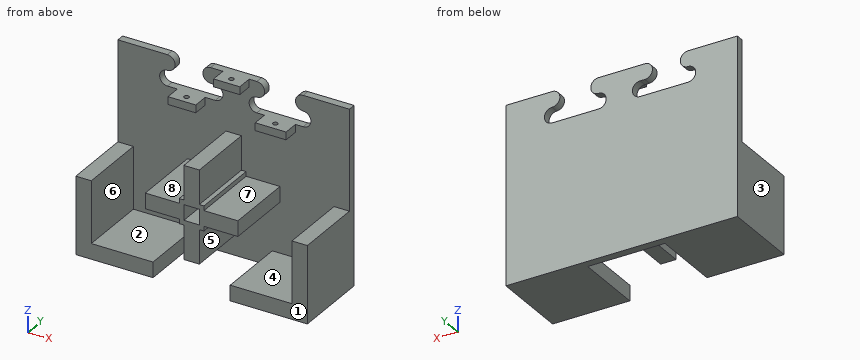
Autodesk Inventor part; units mm, degrees
ref_plane "YZ Plane" through (0, 0, 0) normal (1, 0, 0) x (0, 1, 0)
ref_plane "XZ Plane" through (0, 0, 0) normal (0, 1, 0) x (-1, 0, 0)
ref_plane "XY Plane" through (0, 0, 0) normal (0, 0, 1) x (1, 0, 0)
sketch "puzzle" plane through (0, 0, 0) normal (0, 1, 0) x (-1, 0, 0)
  line L0 (0, -115) -> (-15, -115)
  line L1 (-135, -115) -> (-125, -115)
  line L2 (-135, -115) -> (-150, -115)
  line L3 (-75, -115) -> (-65, -115)
  line L4 (-75, -115) -> (-85.0002, -115)
  line L5 (-105, -135) -> (-94.9796, -135)
  line L6 (-94.9796, -135) -> (-115, -135)
  line L7 (-65, -115) -> (-60, -115)
  line L8 (-60, -125) -> (-63, -125)
  arc A0 (-60, -125) -> (-60, -115) centre (-60, -120) ccw
  arc A1 (-63, -125) -> (-63, -135) centre (-63, -130) ccw
  line L9 (-85.0002, -115) -> (-90.0002, -115)
  line L10 (-94.9796, -135) -> (-89.9796, -135)
  arc A2 (-90.0002, -115) -> (-90, -125) centre (-90.0002, -120) ccw
  arc A3 (-89.9796, -135) -> (-90, -125) centre (-89.9796, -130) ccw
  line L11 (-115, -135) -> (-120, -135)
  line L12 (-125, -115) -> (-120, -115)
  arc A4 (-120, -125) -> (-120, -115) centre (-120, -120) ccw
  arc A5 (-120, -125) -> (-120, -135) centre (-120, -130) ccw
  line L13 (0, -115) -> (-30, -115)
  line L14 (-63, -135) -> (-32.98, -135)
  line L15 (-32.98, -135) -> (-32, -135)
  line L16 (-30, -115) -> (-32, -115)
  arc A6 (-32, -115) -> (-32, -125) centre (-32, -120) ccw
  arc A7 (-32, -135) -> (-32, -125) centre (-32, -130) ccw
  line L17 (0, -115) -> (0, -230)
  line L18 (0, -230) -> (-150, -230)
  line L19 (-150, -230) -> (-150, -115)
  point P0 (0, 0)
  dimension "d22" = 5
  dimension "d23" = 5
  dimension "d24" = 5
  dimension "d25" = 5
  dimension "d26" = 5
  dimension "d76" = 115
extrude "Extrusión4" add sketch "puzzle" along normal blind 5
sketch "Boceto4" plane through (0, 0, 0) normal (0, -1, 0) x (1, 0, 0)
  line L0 (0, -115) -> (0, -230)
  line L1 (32, -115) -> (0, -115)
  line L2 (0, -230) -> (10, -230)
  line L3 (150, -230) -> (0, -230)
  line L4 (10, -180) -> (0, -180)
  line L5 (0, -230) -> (0, -180)
  line L6 (10, -230) -> (50, -230)
  line L7 (50, -230) -> (50, -220)
  line L8 (50, -220) -> (10, -220)
  line L9 (10, -220) -> (10, -180)
  line L10 (150, -230) -> (100, -230)
  line L11 (100, -230) -> (100, -220)
  line L12 (100, -220) -> (140, -220)
  line L13 (140, -220) -> (140, -180)
  line L14 (140, -180) -> (150, -180)
  line L15 (150, -115) -> (150, -230)
  line L16 (150, -230) -> (150, -180)
  line L17 (70, -212.5) -> (80, -212.5)
  line L18 (80, -152.5) -> (70, -152.5)
  line L19 (45, -177.5) -> (45, -187.5)
  line L20 (105, -177.5) -> (105, -187.5)
  line L21 (83, -177.5) -> (83, -174.5)
  line L22 (83, -174.5) -> (80, -174.5)
  line L23 (80, -174.5) -> (80, -152.5)
  line L24 (83, -177.5) -> (105, -177.5)
  line L25 (80, -177.5) -> (80, -187.5)
  line L26 (80, -177.5) -> (70, -177.5)
  line L27 (67, -177.5) -> (67, -174.5)
  line L28 (67, -174.5) -> (70, -174.5)
  line L29 (67, -187.5) -> (67, -190.5)
  line L30 (67, -190.5) -> (70, -190.5)
  line L31 (67, -177.5) -> (45, -177.5)
  line L32 (67, -187.5) -> (45, -187.5)
  line L33 (70, -174.5) -> (70, -152.5)
  line L34 (70, -177.5) -> (70, -182.5)
  line L35 (70, -190.5) -> (70, -212.5)
  line L36 (80, -187.5) -> (70, -187.5)
  line L37 (70, -187.5) -> (70, -182.5)
  line L38 (80, -190.5) -> (83, -190.5)
  line L39 (83, -190.5) -> (83, -187.5)
  line L40 (80, -190.5) -> (80, -212.5)
  line L41 (83, -187.5) -> (105, -187.5)
  point P0 (0, 0)
extrude "Extrusión5" add sketch "Boceto4" along normal blind 45
sketch "Boceto5" plane through (0, 0, 0) normal (0, -1, 0) x (1, 0, 0)
  line L0 (85, -115) -> (68, -115)
  line L1 (68, -120) -> (85, -120)
  line L2 (68, -120) -> (68, -115)
  line L3 (85, -120) -> (85, -115)
  line L4 (32, -135) -> (63, -135)
  line L5 (47.5, -135) -> (38.5, -135)
  line L6 (38.5, -135) -> (56.5, -135)
  line L7 (56.5, -135) -> (56.5, -140)
  line L8 (56.5, -140) -> (38.5, -140)
  line L9 (38.5, -140) -> (38.5, -135)
  line L10 (120, -135) -> (89.9796, -135)
  line L11 (104.9898, -135) -> (94.9898, -135)
  line L12 (94.9898, -135) -> (104.9898, -135)
  line L13 (104.9898, -135) -> (114.9898, -135)
  line L14 (114.9898, -135) -> (114.9898, -140)
  line L15 (114.9898, -140) -> (94.9898, -140)
  line L16 (94.9898, -140) -> (94.9898, -135)
  point P0 (0, 0)
extrude "Extrusión6" add sketch "Boceto5" along normal blind 10
sketch "Boceto6" plane through (89.9796, 5, -135) normal (0, 0, 1) x (1, 0, 0)
  line L0 (10.0204, -5) -> (50.0204, -5)
  line L1 (25, -5) -> (15, -5)
  line L2 (25.0102, -5) -> (25.0102, -15)
  line L3 (25.0102, -5) -> (25.0102, -15)
  line L4 (25.0102, -15) -> (5.0102, -15)
  line L5 (25.0102, -15) -> (5.0102, -15)
  line L6 (15.0204, -5) -> (15.0204, -50)
  circle A0 centre (15.0204, -10) radius 1.6
  line L7 (-33.4796, -15) -> (-51.4796, -15)
  line L8 (-33.4796, -15) -> (-51.4796, -15)
  circle A1 centre (-42.4796, -10) radius 1.6
  point P0 (-89.9796, -5)
  dimension "d120" = 10
  dimension "d121" = 3.2
  dimension "d123" = 3.2
extrude "Extrusión7" cut sketch "Boceto6" against normal blind 10 contours A0 L6 | L6 A0 | A1
sketch "Boceto7" plane through (32, 5, -135) normal (0, 0, 1) x (1, 0, 0)
  circle A0 centre (15.5, -10) radius 1.6
  circle A1 centre (15.5, -10) radius 1.6
  point P0 (-32, -5)
extrude "Extrusión8" cut sketch "Boceto7" against normal blind 34
sketch "Boceto8" plane through (68, 0, -115) normal (0, 0, 1) x (1, 0, 0)
  line L0 (22.0002, 0) -> (-8, 0)
  line L1 (17, 0) -> (0, 0)
  line L2 (0, 0) -> (0, -10)
  line L3 (0, -10) -> (17, -10)
  line L4 (17, -10) -> (17, 0)
  circle A0 centre (8.5, -5) radius 1.6
  point P0 (-68, 0)
  dimension "d128" = 3.2
extrude "Extrusión9" cut sketch "Boceto8" against normal blind 5 contours A0
properties part number "base auxiliar 2"
Source: CAD feature listing. Evaluate the final solid. Frame: model axes, mm. Face numbers are marked on the shaded views. A direction names the side the tool comes from. Coordinates: 2 decimals unless noted, no trailing zeros. Loops run counter-clockwise (first coordinate to the right, second up) from the corner with the lowest first, then second, coordinate; pieces in that order, holes last. Notation, with made-up numbers: (56, 10.5) -> (107, 10.5) arc R26 ccw to (107, 48.5) -> close; hole circle Ø8 at (12.25, -9.75). An arc over 180 degrees is marked (long way). Answer in a Markdown table with one row per item. Add a question column.
Q1. Section A-A on z = -130. Return the cut outline in (x, y), and give its area (3 significant figures).
Q2. Section B-B on y = -22. Give the number of separate pieces and of enclosed holes in the cut face, and give its area (3 significant figures).
Q3. Contact query for flat-ended pins moving along their axis: pin 1 Ø5 at (x, y) = (20.5, -19.5) entering from +Z; pin 2 Ø3 at (y, z) = (-4, -157) entering from -X; pin 3 Ø4 at (y, z) = (-31.5, -174.5) entering from -X. Output: stop coordinate, or through.
Q4. Section D-D on y = 2.5. Return the cut outline in (x, z), and give its area (3 significant figures).
Q5. Ray query, line 1 along X through (y, z) = (-5.5, -197); line 2 along Z through (x, y) = (52, -3); line 3 along X through (y, z) = (-21, -179). Return the intervals inside material, ascending.
Q6. Reachability of the marked faces 4, 5, 6, 7 and 8 from +Z, -Z, +X, -X, +Y, -Y: full face, straight path, thin tool, end or side. Return the list, or none.
Q7. Section C-C on x = 108.5. Return the cut outline in (y, z), and give its area (3 significant figures).
Q8. Pull-direction query (X, two-part tool) for the marked faces 1, 2 and 3; classes: pulls with the +X half, pulls with the -X half, needs draft (parallel to the pull), parting line crosses it, or undercut.
Computed values:
| question | item | result |
|---|---|---|
| 1 | outline | (0, 0) -> (27, 0) -> (27, 5) -> (0, 5) -> close; (68, 0) -> (84.98, 0) -> (84.98, 5) -> (68, 5) -> close; (125, 0) -> (150, 0) -> (150, 5) -> (125, 5) -> close |
| 1 | area | 345 mm^2 |
| 2 | separate pieces | 3 |
| 2 | enclosed holes | 1 |
| 2 | area | 2,840 mm^2 |
| 3 | pin 1 | stops at z = -220 |
| 3 | pin 2 | stops at x = 70 |
| 3 | pin 3 | stops at x = 67 |
| 4 | outline | (0, -230) -> (150, -230) -> (150, -115) -> (120, -115) arc R5 ccw to (120, -125) arc R5 cw to (120, -135) -> (89.98, -135) arc R5 cw to (90, -125) arc R5 ccw to (90, -115) -> (60, -115) arc R5 ccw to (60, -125) -> (63, -125) arc R5 cw to (63, -135) -> (32, -135) arc R5 cw to (32, -125) arc R5 ccw to (32, -115) -> (0, -115) -> close |
| 4 | area | 16,100 mm^2 |
| 5 | line 1 | x = 0 to 10, 70 to 80, 140 to 150 |
| 5 | line 2 | z = -187.5 to -177.5, -140 to -135 |
| 5 | line 3 | x = 45 to 70, 80 to 105 |
| 6 | face 4 | -Y |
| 6 | face 5 | -Z, -Y |
| 6 | face 6 | +Z, -Y |
| 6 | face 7 | +X, -Y |
| 6 | face 8 | -X, -Y |
| 7 | outline | (-45, -230) -> (5, -230) -> (5, -135) -> (-10, -135) -> (-10, -140) -> (0, -140) -> (0, -220) -> (-45, -220) -> close |
| 7 | area | 975 mm^2 |
| 8 | face 1 | needs draft |
| 8 | face 2 | undercut |
| 8 | face 3 | pulls with the -X half |
